The listing builds one solid part. Answer for the finished solid, in the listing's coordinates (mm). A direction names the side the tool comes from. Give positions to 0.01 mm unless a question says otherwise; leave off trailing zeros. Write each loop counter-clockwise with the first axis right and the second up, starting at its lowest first coordinate (ties: lowest second). Pieces come first, ordered by that corner, then holes. Notation, with made-up numbers: M -33,49 L 3,49 A13 ccw 3,55 Z; hole C 8.25,69.25 d5. An arc over 180 degrees is marked long. Return JSON: item names as keys, results as strings.
from build123d import *

# Parameters (mm, degrees)
AUFSATZ_LINEAR_AUSTRAGEN1_DEPTH      = 7.5
AUFSATZ_LINEAR_AUSTRAGEN1_DEPTH_BACK = 14.5
SKIZZE1_R                            = 12.5
SKIZZE1_R_2                          = 1.55
SCHNITT_LINEAR_AUSTRAGEN1_DEPTH      = 4.5
AUFSATZ_LINEAR_AUSTRAGEN2_DEPTH      = 5
SCHNITT_LINEAR_AUSTRAGEN4_DEPTH      = 23.86372673
SCHNITT_LINEAR_AUSTRAGEN4_DEPTH_BACK = 23.86372673
SCHNITT_LINEAR_AUSTRAGEN5_DEPTH      = 10
SCHNITT_LINEAR_AUSTRAGEN5_DEPTH_BACK = 23.86372673
SKIZZE5_OUTSIDE_W                    = 35.898
SKIZZE5_OUTSIDE_H                    = 35.898
SKIZZE5_OUTSIDE_W_2                  = 20
SKIZZE5_OUTSIDE_H_2                  = 30
VERRUNDUNG1_R                        = 1.2
VERRUNDUNG2_R                        = 1


with BuildPart() as part:
    # Skizze1 → Aufsatz-Linear austragen1 (new, two sides: drawn at the far end of the back side and taken through both)
    with BuildSketch(Plane.XY.offset(-AUFSATZ_LINEAR_AUSTRAGEN1_DEPTH_BACK)):
        Circle(SKIZZE1_R)
        with Locations((0, 8)):
            Circle(SKIZZE1_R_2, mode=Mode.SUBTRACT)
        with Locations((0, -8)):
            Circle(SKIZZE1_R_2, mode=Mode.SUBTRACT)
    extrude(amount=AUFSATZ_LINEAR_AUSTRAGEN1_DEPTH + AUFSATZ_LINEAR_AUSTRAGEN1_DEPTH_BACK)

    # Skizze2 → Schnitt-Linear austragen1 (cut)
    with BuildSketch(Plane(origin=(0, 0, -14.5), x_dir=(-1, 0, 0), z_dir=(0, 0, -1))):
        with BuildLine():
            Line((-9, -4), (-9, 4))
            ThreePointArc((-9, 4), (-8.707106781, 4.707106781), (-8, 5))
            Line((-8, 5), (8, 5))
            ThreePointArc((8, 5), (8.707106781, 4.707106781), (9, 4))
            Line((9, 4), (9, -4))
            ThreePointArc((9, -4), (8.707106781, -4.707106781), (8, -5))
            Line((8, -5), (-8, -5))
            ThreePointArc((-8, -5), (-8.707106781, -4.707106781), (-9, -4))
        make_face()
    extrude(amount=-SCHNITT_LINEAR_AUSTRAGEN1_DEPTH, mode=Mode.SUBTRACT)

    # Skizze3 → Aufsatz-Linear austragen2 (add)
    with BuildSketch(Plane.XY.offset(7.5)):
        with BuildLine():
            Line((-8, 5), (8, 5))
            ThreePointArc((8, 5), (8.707106781, 4.707106781), (9, 4))
            Line((9, 4), (9, -4))
            ThreePointArc((9, -4), (8.707106781, -4.707106781), (8, -5))
            Line((8, -5), (-8, -5))
            ThreePointArc((-8, -5), (-8.707106781, -4.707106781), (-9, -4))
            Line((-9, -4), (-9, 4))
            ThreePointArc((-9, 4), (-8.707106781, 4.707106781), (-8, 5))
        make_face()
    extrude(amount=AUFSATZ_LINEAR_AUSTRAGEN2_DEPTH)

    # Skizze4 → Schnitt-Linear austragen4 (cut, two sides: drawn at the far end of the back side and taken through both)
    with BuildSketch(Plane.XY.offset(-SCHNITT_LINEAR_AUSTRAGEN4_DEPTH_BACK)):
        with BuildLine():
            Line((-6.5, -3), (6.5, -3))
            ThreePointArc((6.5, -3), (7.207106781, -2.707106781), (7.5, -2))
            Line((7.5, -2), (7.5, 2))
            ThreePointArc((7.5, 2), (7.207106781, 2.707106781), (6.5, 3))
            Line((6.5, 3), (-6.5, 3))
            ThreePointArc((-6.5, 3), (-7.207106781, 2.707106781), (-7.5, 2))
            Line((-7.5, 2), (-7.5, -2))
            ThreePointArc((-7.5, -2), (-7.207106781, -2.707106781), (-6.5, -3))
        make_face()
    extrude(amount=SCHNITT_LINEAR_AUSTRAGEN4_DEPTH + SCHNITT_LINEAR_AUSTRAGEN4_DEPTH_BACK, mode=Mode.SUBTRACT)

    # Skizze5 outside → Schnitt-Linear austragen5 (cut, two sides: drawn at the far end of the back side and taken through both)
    with BuildSketch(Plane.XY.offset(-SCHNITT_LINEAR_AUSTRAGEN5_DEPTH_BACK)):
        Rectangle(SKIZZE5_OUTSIDE_W, SKIZZE5_OUTSIDE_H)
        Rectangle(SKIZZE5_OUTSIDE_W_2, SKIZZE5_OUTSIDE_H_2, mode=Mode.SUBTRACT)
    extrude(amount=SCHNITT_LINEAR_AUSTRAGEN5_DEPTH + SCHNITT_LINEAR_AUSTRAGEN5_DEPTH_BACK, mode=Mode.SUBTRACT)

    # Verrundung1
    verrundung1_edges = [part.edges().sort_by_distance(p)[0] for p in [
        (-8.707106781, 4.707106781, -14.5),
        (-8.707106781, -4.707106781, -14.5),
        (0, -5, -14.5),
        (8.707106781, -4.707106781, -14.5),
        (8.707106781, 4.707106781, -14.5),
        (0, 5, -14.5),
    ]]
    fillet(verrundung1_edges, radius=VERRUNDUNG1_R)

    # Verrundung2
    verrundung2_edges = [part.edges().sort_by_distance(p)[0] for p in [
        (8.707106781, 4.707106781, 7.5),
        (0, 5, 7.5),
        (-8.707106781, 4.707106781, 7.5),
        (-9, 0, 7.5),
        (-8.707106781, -4.707106781, 7.5),
        (0, -5, 7.5),
        (8.707106781, -4.707106781, 7.5),
        (9, 0, 7.5),
    ]]
    fillet(verrundung2_edges, radius=VERRUNDUNG2_R - 0.0001)  # a hair under: the kernel refuses the full size


solid = part.part
Item 1: Which of the six approach directions +Z, -Z, +X, -X, +Y, -Y give full straight-line access (tool end or side, diameter ignored) to faces 1 (the cylindrical face through (8.699, -4.715, -11.682)), 2 (the cylindrical face through (7.199, -2.715, 1.092)), 3 (the cylindrical face through (8.715, -4.699, 10.472))?
Geometry results:
{"face 1": "-Z", "face 2": "+Z, -Z", "face 3": "+Z, +X, -Y"}
Item 2: A cutting plane is placed at D-D, the plane x = 6. Write down the section's boundary in (y, z).
Geometry results:
{"outline": "M -10.97,-14.5 L -6.2,-14.5 A1.2 ccw -5,-13.3 L -5,-10 L -3,-10 L -3,12.5 L -5,12.5 L -5,8.5 A1 cw -6,7.5 L -10.97,7.5 Z; M 3,-10 L 5,-10 L 5,-13.3 A1.2 ccw 6.2,-14.5 L 10.97,-14.5 L 10.97,7.5 L 6,7.5 A1 cw 5,8.5 L 5,12.5 L 3,12.5 Z"}
Item 3: Determine the mould class of faces 4 (the flat face through (0, -3, 1)), 5 (the flat face through (0, -5, 10)), 6 (the cylindrical face through (-0.2, -12.5, -3.7)) for opening direction X: +X half, -X half, draft (parallel to the pull), parting line (faces both ways), or undercut.
Geometry results:
{"face 4": "undercut", "face 5": "draft", "face 6": "parting line"}
Item 4: A cutting plane is placed at B-B, the plane x = 0. Write down the section's boundary in (y, z), plus the area to 3 significant figures.
Geometry results:
{"outline": "M -12.5,-14.5 L -9.55,-14.5 L -9.55,7.5 L -12.5,7.5 Z; M -6.45,-14.5 L -6.2,-14.5 A1.2 ccw -5,-13.3 L -5,-10 L -3,-10 L -3,12.5 L -5,12.5 L -5,8.5 A1 cw -6,7.5 L -6.45,7.5 Z; M 3,-10 L 5,-10 L 5,-13.3 A1.2 ccw 6.2,-14.5 L 6.45,-14.5 L 6.45,7.5 L 6,7.5 A1 cw 5,8.5 L 5,12.5 L 3,12.5 Z; M 9.55,-14.5 L 12.5,-14.5 L 12.5,7.5 L 9.55,7.5 Z", "area": "283 mm2"}
Item 5: Find the intervals of material crossed by line 1 (Y direction, x = 1.25, z = -7.5); line 2 (Y direction, x = 3.75, z = 10.25); line 3 (Z direction, x = -2, y = -11), in increasing order.
Geometry results:
{"line 1": "y = -12.44 to -8.92, -7.08 to -3, 3 to 7.08, 8.92 to 12.44", "line 2": "y = -5 to -3, 3 to 5", "line 3": "z = -14.5 to 7.5"}
Item 6: Given pin 1 Ø1.2 at (y, z) = (-1, 11) entering from -X; pin 2 Ø3 at (x, y) = (0, -8) entering from +Z; pin 3 Ø1 at (x, z) = (1, -12) entering from -Y; pin 4 Ø1.5 at (x, y) = (-6, -9.5) entering from +Z, each flat-ended and moving along its own axis, determine where each tip first touches the part or whether it passes through.
Geometry results:
{"pin 1": "stops at x = -9", "pin 2": "passes through", "pin 3": "stops at y = -12.49", "pin 4": "stops at z = 7.5"}
Item 7: A cutting plane is placed at A-A, the plane z = -12.5. Write down the section's boundary in (x, y), plus the area to 3 significant figures.
Geometry results:
{"outline": "M -10,-7.5 A12.5 ccw 10,-7.5 L 10,7.5 A12.5 ccw -10,7.5 Z; hole M -9,-4 A1 ccw -8,-5 L 8,-5 A1 ccw 9,-4 L 9,4 A1 ccw 8,5 L -8,5 A1 ccw -9,4 Z; hole C 0,-8 d3.1; hole C 0,8 d3.1", "area": "246 mm2"}
Item 8: A cutting plane is placed at C-C, the plane y = 8.5. Write down the section's boundary in (x, z).
Geometry results:
{"outline": "M -9.17,-14.5 L -1.47,-14.5 L -1.47,7.5 L -9.17,7.5 Z; M 1.47,-14.5 L 9.17,-14.5 L 9.17,7.5 L 1.47,7.5 Z"}
